from build123d import *

# Parameters (mm, degrees)
SKETCH2_R               = 14.7701
SKETCH2_R_2             = 13.3223
SKETCH7_R               = 3.175
CUT_EXTRUDE1_DEPTH      = 31.75
CUT_EXTRUDE2_DEPTH      = 2746.095657429
CUT_EXTRUDE2_DEPTH_BACK = 2746.095657429
SKETCH8_R               = 3.175


with BuildPart() as part:
    # Sweep1: sweep along a path in Sketch1
    with BuildLine(Plane.XY) as sweep1_path:
        Line((0, 0), (0, 1219.2))
        ThreePointArc((0, 1219.2), (-240.237739707, 2036.774718578), (-884.574102374, 2594.424468676))
    # Sketch2 → Sweep1 (sweep)
    with BuildSketch(Plane(origin=(0, 0, 0), x_dir=(1, 0, 0), z_dir=(0, 1, 0))):
        with Locations((-14.7701, 0)):
            Circle(SKETCH2_R)
        with Locations((-14.7701, 0)):
            Circle(SKETCH2_R_2, mode=Mode.SUBTRACT)
    sweep(path=sweep1_path.line)

    # Sketch7 → Cut-Extrude1 (cut)
    with BuildSketch(Plane(origin=(0, 0, 0), x_dir=(0, 0, -1), z_dir=(1, 0, 0))):
        with Locations((0, 304.8)):
            Circle(SKETCH7_R)
        with Locations((0, 1193.8)):
            Circle(SKETCH7_R)
    extrude(amount=-CUT_EXTRUDE1_DEPTH, mode=Mode.SUBTRACT)

    # Sketch8 → Cut-Extrude2 (cut, two sides: drawn at the far end of the back side and taken through both)
    with BuildSketch(Plane.XY.offset(-CUT_EXTRUDE2_DEPTH_BACK)):
        with Locations(Location((-867.881837823, 2569.802206518, 0), (0, 0, 343.480242045))):
            Circle(SKETCH8_R)
        with Locations(Location((-845.023200114, 2558.710815323, 0), (0, 0, 341.89235985))):
            Circle(SKETCH8_R)
    extrude(amount=CUT_EXTRUDE2_DEPTH + CUT_EXTRUDE2_DEPTH_BACK, mode=Mode.SUBTRACT)


solid = part.part
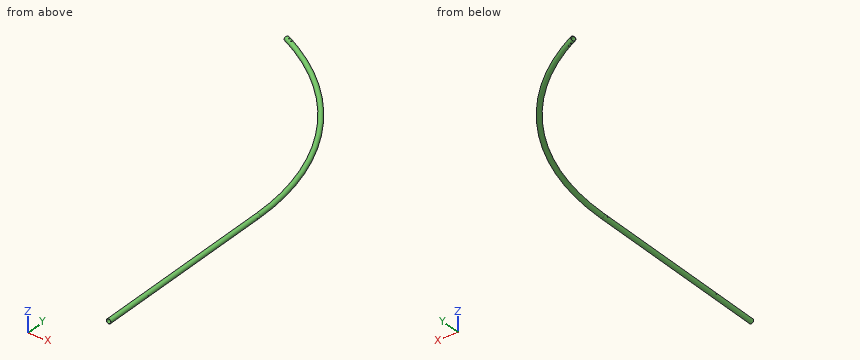
Input: part model. Units: mm. Frame: model coordinates. Give positions to 0.01 mm unless a question says otherwise; leave off trailing zeros. Order: outer loops, then holes, each group sorted by start corner. A loop starts at its lowest first (then second) coordinate and runs counter-clockwise, first axis right, second up.
Q1. Section A-A on y = 589.5. Output: boundary loops of the cut face in (x, z).
Checked values:
outline: circle Ø29.54 at (-14.77, 0); hole circle Ø26.64 at (-14.77, 0)
Q2. Contact query for flat-ended pins moving along their axis: pin 1 Ø3 at (x, z) = (-163, -8) entering from +Y; pin 2 Ø8 at (y, z) = (2185, 4.5) entering from -X; pin 3 Ø3 at (y, z) = (1735.5, 9) entering from +X; pin 4 Ø4 at (y, z) = (304.8, 0) entering from -X (1 decimal). Output: stop coordinate, or through.
Checked values:
pin 1: stops at y = 1900.28
pin 2: stops at x = -390.34
pin 3: stops at x = -92.96
pin 4: passes through
Q3. Ray query, probe 1 along X at (y, z) = (2056.5, -10); probe 2 along X at (y, z) = (1949, -3.5); probe 3 along Y at (x, z) = (-757.5, 10.5). Return the intervals inside material, ascending.
Checked values:
probe 1: x = -284.06 to -281.56, -260.32 to -257.83
probe 2: x = -221.24 to -219.52, -190.08 to -188.37
probe 3: y = 2499.98 to 2502.52, 2521.5 to 2524.03
